Verification items for the finished model (mm, model axes). A direction names the side the tool comes from. Give positions to 0.01 mm unless a question says otherwise; leave off trailing zeros. Write each loop counter-clockwise with the first axis right and the second up, starting at its lowest first coordinate (ties: lowest second). Pieces come first, ordered by that corner, then holes. Notation, with made-up numbers: (74.25, -23.5) -> (93.25, -23.5) arc R20 ccw to (93.25, 2.5) -> close; hole circle Ø7 at (25.5, 45). An arc over 180 degrees is marked (long way). Use one line per item in the form item = value. Start each with the question number.
(1) Section check B-B, the plane y = 66.5. Record the cut outline in (x, z).
(2) Set-up check for faces 1 (the face through (-85.374, 46.203, 2.465)), 2 (the face through (-62.86, 105.39, 2.46)): record each of +Z, -Z, +X, -X, +Y, -Y from which the full face is reachable in a straight line by a thin tool's end or side.
(3) Section check A-A, the plane x = 93. Record the cut outline in (y, z).
(4) Section check D-D, the plane x = -29.5. Record the cut outline in (y, z) (3 decimals), plus the area to 3 significant figures.
(5) Scan lines: L1, parallel to X at y = 123, z = 1.7; L2, parallel to Y at x = -90.5, z = 2.25 (3 decimals); L3, parallel to Y at x = -92, z = 1.6. Record each from-to range of solid material in increasing order.
(6) Release check for a two-part mould opening along X. For faces 3 (the face through (-49.3, 122.815, 2.465)), 4 (the face through (60.72, 108.32, 2.46)), 5 (the face through (100, 49, 2)) record: pulls with the +X half, pulls with the -X half, needs draft (parallel to the pull), parting line crosses it, or undercut.
(7) Section check C-C, the plane z = 2.4. State how many separate pieces and enclosed holes the cut face has, plus the area to 3 significant figures.
(8) Depth check by flat-ended pin: pin 1 Ø1 at (x, z) = (11.5, 0.5) entering from +Y; pin 2 Ø1 at (x, z) = (49, 3) entering from +Y (3 decimals); pin 3 Ø1 at (x, z) = (-47.5, 1.5) entering from -Y. Enter the tip coordinate at first touch or a pass-through.
from build123d import *

# Parameters (mm, degrees)
F0_R     = 5
F1_DEPTH = 5


with BuildPart() as f1:
    # F0 (on Top) → F1 (new body)
    with BuildSketch(Plane.XY):
        Polygon((80.628272, 93.717277), (90, 0), (100, 0), (100, 100), (80, 100), align=None)
        with Locations((93, 39)):
            Circle(F0_R, mode=Mode.SUBTRACT)
        with Locations((92, 54)):
            Circle(F0_R, mode=Mode.SUBTRACT)
        with Locations((92, 69)):
            Circle(F0_R, mode=Mode.SUBTRACT)
        with Locations((92, 84)):
            Circle(F0_R, mode=Mode.SUBTRACT)
        Polygon((-100, 0), (-90, 0), (-80.61579, 93.717277), (-80.000474, 99.86225), (-100, 100), align=None)
        with Locations((-93.288932, 39)):
            Circle(F0_R, mode=Mode.SUBTRACT)
        with Locations((-92, 53.944519)):
            Circle(F0_R, mode=Mode.SUBTRACT)
        with Locations((-92, 68.944519)):
            Circle(F0_R, mode=Mode.SUBTRACT)
        with Locations((-92, 83.944519)):
            Circle(F0_R, mode=Mode.SUBTRACT)
        Polygon((0, 145), (0, 130), (80.628272, 93.717277), (80, 100), (100, 100), align=None)
        with Locations((65.71529, 108.104219)):
            Circle(F0_R, mode=Mode.SUBTRACT)
        with Locations((47.47686, 116.311512)):
            Circle(F0_R, mode=Mode.SUBTRACT)
        with Locations((29.23843, 124.518806)):
            Circle(F0_R, mode=Mode.SUBTRACT)
        with Locations((11, 132.726099)):
            Circle(F0_R, mode=Mode.SUBTRACT)
        Polygon((-80.61579, 93.717277), (0, 130), (0, 145), (-100, 100), (-80.000474, 99.86225), align=None)
        with Locations((-67.475909, 107.307439)):
            Circle(F0_R, mode=Mode.SUBTRACT)
        with Locations((-49.237955, 115.515789)):
            Circle(F0_R, mode=Mode.SUBTRACT)
        with Locations((-29.237955, 124.517183)):
            Circle(F0_R, mode=Mode.SUBTRACT)
        with Locations((-11, 132.725533)):
            Circle(F0_R, mode=Mode.SUBTRACT)
    extrude(amount=F1_DEPTH)


solid = f1.part
Completed:
q1.outline = (-100, 0) -> (-96.36, 0) -> (-96.36, 5) -> (-100, 5) -> close; (-87.64, 0) -> (-83.34, 0) -> (-83.34, 5) -> (-87.64, 5) -> close; (83.35, 0) -> (87.67, 0) -> (87.67, 5) -> (83.35, 5) -> close; (96.33, 0) -> (100, 0) -> (100, 5) -> (96.33, 5) -> close
q2.face_1 = +Z, -Z, -Y
q2.face_2 = +Z, -Z
q3.outline = (0, 0) -> (34, 0) -> (34, 5) -> (0, 5) -> close; (44, 0) -> (49.1, 0) -> (49.1, 5) -> (44, 5) -> close; (58.9, 0) -> (64.1, 0) -> (64.1, 5) -> (58.9, 5) -> close; (73.9, 0) -> (79.1, 0) -> (79.1, 5) -> (73.9, 5) -> close; (88.9, 0) -> (103.15, 0) -> (103.15, 5) -> (88.9, 5) -> close
q4.outline = (116.723, 0) -> (119.524, 0) -> (119.524, 5) -> (116.723, 5) -> close; (129.51, 0) -> (131.725, 0) -> (131.725, 5) -> (129.51, 5) -> close
q4.area = 25.1 mm²
q5.L1 = -48.89 to -34, -24.47 to -15.55, 15.56 to 24.47, 34 to 48.89
q5.L2 = 0 to 34.85, 43.15 to 49.175, 58.714 to 64.175, 73.714 to 79.175, 88.714 to 104.275
q5.L3 = 0 to 34.17, 43.83 to 48.94, 58.94 to 63.94, 73.94 to 78.94, 88.94 to 103.6
q6.face_3 = pulls with the -X half
q6.face_4 = undercut
q6.face_5 = pulls with the +X half
q7.separate_pieces = 1
q7.enclosed_holes = 16
q7.area = 4,330 mm²
q8.pin_1 = 140.05
q8.pin_2 = 123.175
q8.pin_3 = 108.4
